Autodesk Inventor part; units mm, degrees
ref_plane "YZ Plane" through (0, 0, 0) normal (1, 0, 0) x (0, 1, 0)
ref_plane "XZ Plane" through (0, 0, 0) normal (0, 1, 0) x (-1, 0, 0)
ref_plane "XY Plane" through (0, 0, 0) normal (0, 0, 1) x (1, 0, 0)
sketch "Boceto1" plane through (0, 0, 0) normal (1, 0, 0) x (0, 1, 0)
  arc A0 (4.672, 23.7647) -> (-4.8784, 16.507) centre (0, 20) ccw
  arc A1 (15.5865, -12.0751) -> (26.7286, -3.6079) centre (21.278, -8) ccw
  line L0 (26.7286, -3.6079) -> (4.672, 23.7647)
  line L1 (-4.8784, 16.507) -> (15.5865, -12.0751)
  arc A2 (14.7734, -12.6573) -> (27.5073, -2.9805) centre (21.278, -8) ccw
  arc A3 (5.4506, 24.3921) -> (-5.6915, 15.9249) centre (0, 20) ccw
  line L2 (27.5073, -2.9805) -> (5.4506, 24.3921)
  line L3 (-5.6915, 15.9249) -> (14.7734, -12.6573)
  point P0 (0, 0)
  dimension "d2" = 6
  dimension "d3" = 7
  dimension "d4" = 8
  dimension "d5" = 20
  dimension "d6" = 3.259
  dimension "d7" = 16
  dimension "d8" = 14
extrude "Extrusión1" add sketch "Boceto1" along normal blind 16
properties part number "banda"
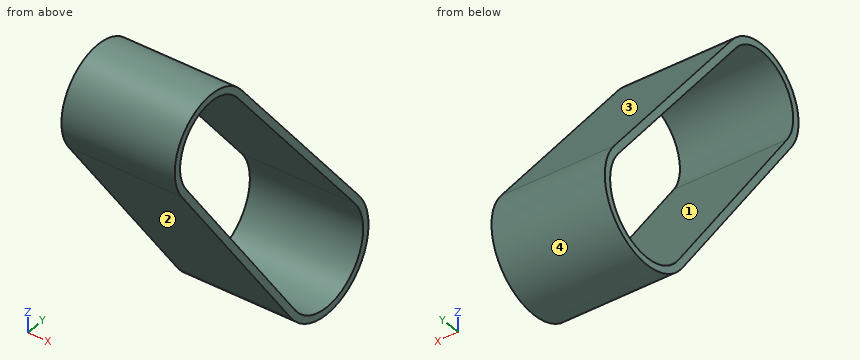
Can you work these out from the model? Positions are in its coordinate system, mm. Face numbers are marked on the shaded views. Coordinates: 2 decimals unless noted, no trailing zeros. Order: outer loops, then holes, each group sorted by start corner. A loop starts at its lowest first (then second) coordinate and runs counter-clockwise, first axis right, second up. Notation, with made-up numbers: (-15, 21.25) -> (28, 21.25) arc R21 ccw to (28, 54.25) -> close; hole circle Ø2 at (74, 60). An arc over 180 degrees is marked (long way). Use one line per item in the form item = value.
Q1. Will these pins go through, and if not, where does the flat tip stop? P1, Ø3, axis at x = 5.5, z = -6, coming from the +Y side; P2, Ø3, axis at x = 9, z = 19.5, coming from the +Y side; P3, Ø10, axis at y = 17, z = -4.5, coming from the -X side; P4, Ø1.5, axis at x = 6.5, y = -1.5, coming from the -Z side.
From the geometry:
P1 = 29.26
P2 = 10.6
P3 = through
P4 = 9.02
Q2. Imagine slicing it at C-C, the plane y = 7.5. List the corners of the cut face in (x, z) for me.
From the geometry:
outline = (0, -2.5) -> (16, -2.5) -> (16, -0.78) -> (0, -0.78) -> close; (0, 20.26) -> (16, 20.26) -> (16, 21.85) -> (0, 21.85) -> close
Q3. We'd pull the mould along Z, two halves only. Please class the marked faces 1, 2, 3 and 4: released by +Z, released by -Z, zero draft, split by the parting line, or undercut.
From the geometry:
face_1 = undercut
face_2 = released by -Z
face_3 = released by +Z
face_4 = split by the parting line
Q4. Imagine slicing it at B-B, the plane z = -8. List the corners of the cut face in (x, y) for me.
From the geometry:
outline = (0, 11.44) -> (16, 11.44) -> (16, 12.67) -> (0, 12.67) -> close; (0, 28.28) -> (16, 28.28) -> (16, 29.28) -> (0, 29.28) -> close
Q5. I need wall thicknesses on L1, parallel to Y at x = 14.5, z = 15; L2, parallel to Y at x = 8.75, z = 1; L3, parallel to Z at x = 10, y = 10. Which ranges of each line are inside material? Lowest first, please.
From the geometry:
L1 = -5.03 to -3.8, 11.73 to 13.02
L2 = 4.99 to 6.22, 23.02 to 24.3
L3 = -5.99 to -4.27, 17.15 to 18.75
